The model under review builds one solid part; all positions refer to its coordinate system, in mm. A direction names the side the tool comes from. Round coordinates to 2 decimals unless told otherwise and drop trailing zeros. Write each loop counter-clockwise with the first axis right and the second up, starting at its lowest first coordinate (ties: lowest second). Pieces come first, ordered by that corner, then holes. Notation, with made-up numbers: M 77,-33 L 102,-33 A25 ccw 102,2 Z; hole C 82.5,51 d2. An arc over 180 degrees is marked long. Write item = value, one per line. Start each with the question number.
Item 1: For pin 1 Ø1.6 at (x, z) = (-1.9, 22.35) entering from +Y, flat-tipped, find the tip position at first contact; note if it passes through.
Item 2: To check wall thickness, follow line 1 along Z through (x, y) = (-1.9, -0.6); line 2 along Z through (x, y) = (-0.6, -0.25); line 3 along X through (y, z) = (-0.25, 22.35). State the ranges of each line that lie inside material, in increasing order.
Item 3: Take a section at B-B, the plane y = -0.8. Give the boundary of the cut face in (x, z), plus the area to 3 significant figures.
Item 4: Take a section at A-A, the plane x = -0.6. Give the boundary of the cut face in (y, z).
Item 5: Tool access review of faces 5 (the flat face through (-0.5, -0.5, 6)), 6 (the flat face through (-2, -1, 13)): name each direction out of +Z, -Z, +X, -X, +Y, -Y from which nothing blocks a thin tool from reaching the whole face with its end or side.
Item 6: Take a section at D-D, the plane x = -1.9. Give the boundary of the cut face in (y, z), plus the area to 3 significant figures.
Item 7: Take a section at C-C, the plane z = 2.65. Give the boundary of the cut face in (x, y), plus the area to 3 significant figures.
Item 8: The part is to be moulded in two halves that separate along Z. For faces 1 (the flat face through (0, -0.5, 22)), 2 (the flat face through (-2, -0.5, 25)), 3 (the flat face through (-1, -0.5, 12.4)), 4 (the flat face through (-2, -0.5, 0)), say which applies: +Z half, -Z half, draft (parallel to the pull), parting line (faces both ways), or undercut.
Autodesk Inventor part; units mm, degrees
ref_plane "YZ Plane" through (0, 0, 0) normal (1, 0, 0) x (0, 1, 0)
ref_plane "XZ Plane" through (0, 0, 0) normal (0, 1, 0) x (-1, 0, 0)
ref_plane "XY Plane" through (0, 0, 0) normal (0, 0, 1) x (1, 0, 0)
sketch "Sketch1" plane through (0, 0, 0) normal (0, 1, 0) x (-1, 0, 0)
  point P0 (0, 0)
sketch "Sketch2" plane through (0, 0, 0) normal (0, 1, 0) x (-1, 0, 0)
  line L0 (0, 0) -> (4, 0)
  line L1 (4, 0) -> (4, 25)
  line L2 (4, 25) -> (0, 25)
  line L3 (0, 25) -> (0, 0)
  point P0 (3, 0)
  point P1 (0, 6)
  point P2 (0, 19)
  dimension "d0" = 4
  dimension "d1" = 25
extrude "Extrusion1" add sketch "Sketch2" against normal blind 1
sketch "Sketch3" plane through (0, 0, 0) normal (0, 1, 0) x (-1, 0, 0)
  line L0 (1, 19) -> (0, 19)
  line L1 (0, 19) -> (0, 6)
  line L2 (0, 6) -> (1, 6)
  line L3 (1, 6) -> (1, 19)
  point P0 (0, 0)
  point P1 (0, 2.65)
  point P2 (0, 0)
  point P3 (0, 22.35)
  point P4 (-6.35, -25.4)
  point P5 (3, 25)
  point P6 (3, 22.35)
  point P7 (3, 2.65)
  dimension "d4" = 13
  dimension "d20" = 1
extrude "Extrusion2" cut sketch "Sketch3" against normal blind 1
sketch "Sketch6" plane through (0, 0, 0) normal (0, 1, 0) x (1, 0, 0)
  point P0 (0, 0)
sketch "Sketch7" plane through (0, 0, 0) normal (0, 1, 0) x (1, 0, 0)
  line L0 (-4, 0) -> (-4, -25)
  line L1 (-4, -25) -> (0, -25)
  point P0 (0, 0)
  point P1 (-1.9, -2.65)
  point P2 (-1.9, -22.35)
  dimension "d21" = 2.1
  dimension "d22" = 2.65
  dimension "d23" = 2.65
  dimension "d24" = 2.1
hole "Hole2" at (-1.9, 0, 2.65) at (-1.9, 0, 22.35) direction (0, -1, 0) diameter 2 depth 2 tip angle 118
properties part number "headplate_ephys"
Response values:
q1.pin_1 = through
q2.line_1 = 0 to 1.65, 3.65 to 21.35, 23.35 to 25
q2.line_2 = 0 to 6, 19 to 25
q2.line_3 = -4 to -2.9, -0.9 to 0
q3.outline = M -4,0 L 0,0 L 0,6 L -1,6 L -1,19 L 0,19 L 0,25 L -4,25 Z; hole C -1.9,2.65 d2; hole C -1.9,22.35 d2
q3.area = 80.7 mm2
q4.outline = M -1,0 L 0,0 L 0,6 L -1,6 Z; M -1,19 L 0,19 L 0,25 L -1,25 Z
q5.face_5 = +X, +Y, -Y
q5.face_6 = +Z, -Z, +X, -X, -Y
q6.outline = M -1,0 L 0,0 L 0,1.65 L -1,1.65 Z; M -1,3.65 L 0,3.65 L 0,21.35 L -1,21.35 Z; M -1,23.35 L 0,23.35 L 0,25 L -1,25 Z
q6.area = 21.0 mm2
q7.outline = M -4,-1 L -2.9,-1 L -2.9,0 L -4,0 Z; M -0.9,-1 L 0,-1 L 0,0 L -0.9,0 Z
q7.area = 2.00 mm2
q8.face_1 = draft
q8.face_2 = +Z half
q8.face_3 = undercut
q8.face_4 = -Z half
